Verification items for the finished model (mm, model axes). A direction names the side the tool comes from. Give positions to 0.01 mm unless a question says otherwise; leave off trailing zeros. Write each loop counter-clockwise with the first axis right and the second up, starting at its lowest first coordinate (ties: lowest second). Pieces come first, ordered by that corner, then holes. Notation, with made-up numbers: M 70,19 L 124,19 A8 ccw 124,32 Z; hole C -3,-33.5 d8. An arc over 180 degrees is marked long. Answer as a JSON object with one key per item and string values.
```python
from build123d import *

# Parameters (mm, degrees)
F1_DEPTH = 12
F2_R     = 2.5
F3_DEPTH = 25


with BuildPart() as f1:
    # F0 (on Front) → F1 (new body)
    with BuildSketch(Plane.XZ):
        with BuildLine():
            ThreePointArc((-4, 4), (0, 8), (4, 4))
            Line((4, 4), (4, 0))
            Line((4, 0), (18, 0))
            Line((18, 0), (18, 0.5))
            Line((18, 0.5), (7, 0.5))
            Line((7, 0.5), (7, 4))
            ThreePointArc((7, 4), (0, 11), (-7, 4))
            Line((-7, 4), (-7, 0.5))
            Line((-7, 0.5), (-18, 0.5))
            Line((-18, 0.5), (-18, 0))
            Line((-18, 0), (-4, 0))
            Line((-4, 0), (-4, 4))
        make_face()
    extrude(amount=F1_DEPTH)

    # F2 (on face) → F3 (cut)
    with BuildSketch(Plane(origin=(0, 0, 0), x_dir=(1, 0, 0), z_dir=(0, 0, -1))):
        with Locations((-13, 6)):
            Circle(F2_R)
        with Locations((13, 6)):
            Circle(F2_R)
        with BuildLine():
            ThreePointArc((-16.970563, 0), (-17.740774, 2.956164), (-18, 6))
            Line((-18, 6), (-18, 0))
            Line((-18, 0), (-16.970563, 0))
        make_face()
        with BuildLine():
            ThreePointArc((-18, 6), (-17.740774, 9.043836), (-16.970563, 12))
            Line((-16.970563, 12), (-18, 12))
            Line((-18, 12), (-18, 6))
        make_face()
        with BuildLine():
            ThreePointArc((16.970563, 12), (17.740774, 9.043836), (18, 6))
            Line((18, 6), (18, 12))
            Line((18, 12), (16.970563, 12))
        make_face()
        with BuildLine():
            Line((16.970563, 0), (18, 0))
            Line((18, 0), (18, 6))
            ThreePointArc((18, 6), (17.740774, 2.956164), (16.970563, 0))
        make_face()
    extrude(amount=-F3_DEPTH, mode=Mode.SUBTRACT)


solid = f1.part
```
1) Section check C-C on z = 5. Record the boundary of the cut face in (x, y), and give its area (3 significant figures).
Completed:
{"outline": "M -6.93,-12 L -3.87,-12 L -3.87,0 L -6.93,0 Z; M 3.87,-12 L 6.93,-12 L 6.93,0 L 3.87,0 Z", "area": "73.3 mm2"}
2) Section check B-B on y = -4.5. Record the boundary of the cut face in (x, z), and give its area (3 significant figures).
Completed:
{"outline": "M -17.94,0 L -15,0 L -15,0.5 L -17.94,0.5 Z; M -11,0 L -4,0 L -4,4 A4 cw 4,4 L 4,0 L 11,0 L 11,0.5 L 7,0.5 L 7,4 A7 ccw -7,4 L -7,0.5 L -11,0.5 Z; M 15,0 L 17.94,0 L 17.94,0.5 L 15,0.5 Z", "area": "82.8 mm2"}
3) Section check D-D on y = -10. Record the boundary of the cut face in (x, z).
Completed:
{"outline": "M -17.55,0 L -4,0 L -4,4 A4 cw 4,4 L 4,0 L 17.55,0 L 17.55,0.5 L 7,0.5 L 7,4 A7 ccw -7,4 L -7,0.5 L -17.55,0.5 Z"}
4) Thickness scan on L1, parallel to X at y = -6, z = 0.25; L2, parallel to X at y = -11, z = 2; L3, parallel to Z at x = -16, y = -4. Record the ranges inside material, lowest first.
Completed:
{"L1": "x = -18 to -15.5, -10.5 to -4, 4 to 10.5, 15.5 to 18", "L2": "x = -7 to -4, 4 to 7", "L3": "z = 0 to 0.5"}
5) Go/stop test with flat-tipped pins: pin 1 (4 mm diameter, centred on x = 12.5, y = -3, fed in from +Z); pin 2 (1.2 mm diameter, centred on y = -6.5, z = 3, fed in from +X); pin 3 (5 mm diameter, centred on x = 11, z = 5.5, fed in from +Y); pin 4 (4 mm diameter, centred on x = 5, y = -10, fed in from +Z). Record where each tip stops, or that it passes through.
Completed:
{"pin 1": "stops at z = 0.5", "pin 2": "stops at x = 7", "pin 3": "passes through", "pin 4": "stops at z = 10.32"}
6) Section check A-A on x = -13. Record the boundary of the cut face in (y, z), and give its area (3 significant figures).
Completed:
{"outline": "M -12,0 L -8.5,0 L -8.5,0.5 L -12,0.5 Z; M -3.5,0 L 0,0 L 0,0.5 L -3.5,0.5 Z", "area": "3.50 mm2"}
7) Release check for a two-part mould opening along X. For faces 1 (the face through (10.5, -6.1, 0.2)), 2 (the face through (10, -6, 0.5)), 3 (the face through (-7, -6, 2)), 4 (the face through (0, -6, 8)) record: pulls with the +X half, pulls with the -X half, needs draft (parallel to the pull), parting line crosses it, or undercut.
Completed:
{"face 1": "undercut", "face 2": "needs draft", "face 3": "pulls with the -X half", "face 4": "undercut"}
8) Access from +Z, -Z, +X, -X, +Y, -Y to the whole of each face (thin tool, end or side, straight path). Record for faces 5 (the face through (7, -6, 2)), 6 (the face through (-1.3, 0, 8)), 7 (the face through (-4, -6, 2)), 8 (the face through (9, -6, 0)), 9 (the face through (-10, -6, 0.5)).
Completed:
{"face 5": "+Z, +X, +Y, -Y", "face 6": "+Z, -Z, +X, -X, +Y", "face 7": "-Z, +Y, -Y", "face 8": "-Z, +X, -X, +Y, -Y", "face 9": "+Z, -X, +Y, -Y"}
